```python
from build123d import *

# Parameters (mm, degrees)
SKETCH1_R                  = 37.5
BOSS_EXTRUDE1_DEPTH        = 250
M8X1_25_TAPPED_HOLE1_D     = 6.8
M8X1_25_TAPPED_HOLE1_DEPTH = 21.25
M8X1_25_TAPPED_HOLE1_TIP   = 2.042926105
M8X1_25_TAPPED_HOLE2_D     = 6.8
M8X1_25_TAPPED_HOLE2_DEPTH = 21.25
M8X1_25_TAPPED_HOLE2_TIP   = 2.042926105
M8X1_25_TAPPED_HOLE3_D     = 6.8
M8X1_25_TAPPED_HOLE3_DEPTH = 21.25
M8X1_25_TAPPED_HOLE3_TIP   = 2.042926105
M8X1_25_TAPPED_HOLE4_D     = 6.8
M8X1_25_TAPPED_HOLE4_DEPTH = 21.25
M8X1_25_TAPPED_HOLE4_TIP   = 2.042926105


with BuildPart() as part:
    # Sketch1 → Boss-Extrude1 (new body, symmetric)
    with BuildSketch(Plane.XY):
        Circle(SKETCH1_R)
    extrude(amount=BOSS_EXTRUDE1_DEPTH, both=True)

    # M8x1.25 Tapped Hole1
    with Locations(Plane(origin=(0, -37.5, 0), x_dir=(-1, 0, 0), z_dir=(0, -1, 0))):
        with Locations((0, 0)):
            Hole(M8X1_25_TAPPED_HOLE1_D / 2, depth=M8X1_25_TAPPED_HOLE1_DEPTH)
            with Locations((0, 0, -(M8X1_25_TAPPED_HOLE1_DEPTH + M8X1_25_TAPPED_HOLE1_TIP / 2))):  # 118° drill point
                Cone(0, M8X1_25_TAPPED_HOLE1_D / 2, M8X1_25_TAPPED_HOLE1_TIP, mode=Mode.SUBTRACT)

    # M8x1.25 Tapped Hole2
    with Locations(Plane(origin=(0, 37.5, 0), x_dir=(1, 0, 0), z_dir=(0, 1, 0))):
        with Locations((0, 0)):
            Hole(M8X1_25_TAPPED_HOLE2_D / 2, depth=M8X1_25_TAPPED_HOLE2_DEPTH)
            with Locations((0, 0, -(M8X1_25_TAPPED_HOLE2_DEPTH + M8X1_25_TAPPED_HOLE2_TIP / 2))):  # 118° drill point
                Cone(0, M8X1_25_TAPPED_HOLE2_D / 2, M8X1_25_TAPPED_HOLE2_TIP, mode=Mode.SUBTRACT)

    # M8x1.25 Tapped Hole3
    with Locations(Plane(origin=(37.5, 0, 0), x_dir=(0, 0, -1), z_dir=(1, 0, 0))):
        with Locations((0, 0)):
            Hole(M8X1_25_TAPPED_HOLE3_D / 2, depth=M8X1_25_TAPPED_HOLE3_DEPTH)
            with Locations((0, 0, -(M8X1_25_TAPPED_HOLE3_DEPTH + M8X1_25_TAPPED_HOLE3_TIP / 2))):  # 118° drill point
                Cone(0, M8X1_25_TAPPED_HOLE3_D / 2, M8X1_25_TAPPED_HOLE3_TIP, mode=Mode.SUBTRACT)

    # M8x1.25 Tapped Hole4
    with Locations(Plane.ZY.offset(37.5)):
        with Locations((0, 0)):
            Hole(M8X1_25_TAPPED_HOLE4_D / 2, depth=M8X1_25_TAPPED_HOLE4_DEPTH)
            with Locations((0, 0, -(M8X1_25_TAPPED_HOLE4_DEPTH + M8X1_25_TAPPED_HOLE4_TIP / 2))):  # 118° drill point
                Cone(0, M8X1_25_TAPPED_HOLE4_D / 2, M8X1_25_TAPPED_HOLE4_TIP, mode=Mode.SUBTRACT)


solid = part.part
```
Work out the finished part from the listing and answer in its coordinate system (mm). Round coordinates to 2 decimals unless told otherwise and drop trailing zeros. Write each loop counter-clockwise with the first axis right and the second up, starting at its lowest first coordinate (ties: lowest second). Pieces come first, ordered by that corner, then holes.
1) Consider probe 1 along Z at (x, y) = (30, 0); probe 2 along X at (y, z) = (-2.5, 179); probe 3 along Z at (x, y) = (20.5, -2). Determine where each line is inside the solid, lowest interval first.
2) Flat-ended cylindrical pins translate along their axes: P1, Ø5.5, axis at x = 0, z = 0, coming from the -Y side; P2, Ø10, axis at x = -26, z = -22.5, coming from the -Y side; P3, Ø5.5, axis at y = 0, z = 0, coming from the +X side. Find the tip coordinate at first contact, or state that the pin passes through.
3) A cutting plane is placed at A-A on z = 24. Determine the outline of the cut face in (x, y), and give its area (3 significant figures).
4) A cutting plane is placed at C-C on x = -9. Determine the outline of the cut face in (y, z).
5) A cutting plane is placed at B-B on x = 10. Determine the outline of the cut face in (y, z).
Entries:
1. probe 1: z = -250 to -3.4, 3.4 to 250
1. probe 2: x = -37.42 to 37.42
1. probe 3: z = -250 to -2.75, 2.75 to 250
2. P1: stops at y = -15.86
2. P2: stops at y = -31.07
2. P3: stops at x = 15.86
3. outline: circle Ø75 at (0, 0)
3. area: 4,420 mm2
4. outline: (-36.4, -250) - (36.4, -250) - (36.4, 250) - (-36.4, 250) - close
5. outline: (-36.14, -250) - (36.14, -250) - (36.14, 250) - (-36.14, 250) - close
